Read the model definition and answer for the solid it produces. Units are mm, in the model's axes. Face numbers are marked on the shaded views. A direction names the side the tool comes from. Coordinates: 2 decimals unless noted, no trailing zeros. Order: outer loops, then holes, each group sorted by start corner. A loop starts at its lowest first (then second) coordinate and runs counter-clockwise, first axis right, second up. Notation, with made-up numbers: (76.25, 20.5) -> (126.25, 20.5) arc R20 cw to (126.25, 32.5) -> close; hole circle Ø10 at (-38, 54.25). An arc over 180 degrees is marked (long way). Answer as a JSON object with one key per item and string values. Group by question number.
1) Determine the mould class of the marked faces 3, 4, 5 and 6 for opening direction Z: released by +Z, released by -Z, zero draft, split by the parting line, or undercut.
2) Section A-A on x = 48 is taken. Determine the outline of the cut face in (y, z), and give its area (3 significant figures).
3) A tool of negligible diameter and unlimited length cuts with its end or side. For the marked faces 1 and 2, from which of +Z, -Z, +X, -X, +Y, -Y can it reach the whole face along a straight path? Write none if from no direction.
4) Section C-C on z = 3 is taken. Determine the outline of the cut face in (x, y), and give its area (3 significant figures).
5) Section B-B on y = 178.5 is taken. Determine the outline of the cut face in (x, z).
6) Given pin 1 (1 mm diameter, centred on y = 180.5, z = -15, fed in from -X); pin 2 (5 mm diameter, centred on y = 31.5, z = 26.5, fed in from +X); pin 3 (8 mm diameter, centred on x = 19, y = 131.5, fed in from +Z); pin 4 (4 mm diameter, centred on x = 12.7, y = 275, fed in from -Z), each flat-ended and moving along its own axis, determine where each tip first touches the part or whether it passes through.
7) Section D-D on x = 29.5 is taken. Determine the outline of the cut face in (y, z), and give its area (3 significant figures).
8) Consider L1, parallel to Y at x = 12.7, z = -11.5; L2, parallel to Z at x = 54, y = 95; L3, parallel to Y at x = 12.7, z = -3.5. Determine where each line is inside the solid, lowest interval first.
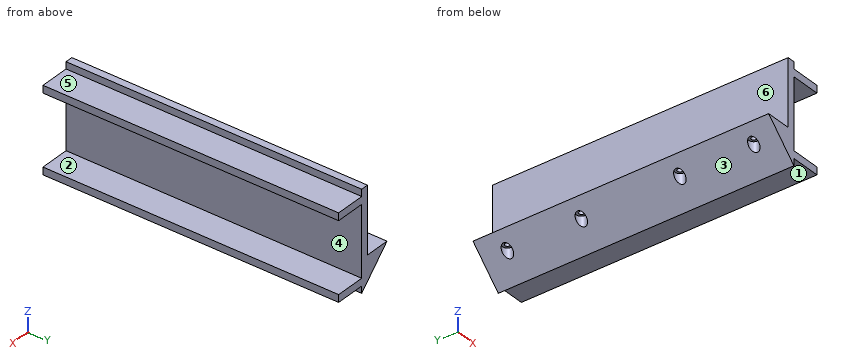
from build123d import *

# Parameters (mm, degrees)
BOSS_EXTRUDE1_DEPTH = 300
SKETCH3_R           = 2.5
CUT_EXTRUDE1_DEPTH  = 51
SKETCH4_R           = 5
CUT_EXTRUDE2_DEPTH  = 19


with BuildPart() as part:
    # Sketch1 → Boss-Extrude1 (new body)
    with BuildSketch(Plane(origin=(0, 0, 0), x_dir=(1, 0, 0), z_dir=(0, 1, 0))):
        Polygon((0, 0), (25.4, 0), (25.4, -50.8), (25.4, -67.1), (32.9, -67.1), (32.9, -60.1), (62.9, -60.1), (62.9, -52.6), (32.9, -52.6), (32.9, 18.4), (62.9, 18.4), (62.9, 25.9), (32.9, 25.9), (32.9, 32.9), align=None)
    extrude(amount=BOSS_EXTRUDE1_DEPTH)

    # Sketch3 → Cut-Extrude1 (cut)
    with BuildSketch(Plane(origin=(-25.9, 0, -25.9), x_dir=(1, 0, 0), z_dir=(0, 0, 1))):
        with Locations((38.6, 275)):
            Circle(SKETCH3_R)
        with Locations((38.6, 200)):
            Circle(SKETCH3_R)
        with Locations((38.6, 100)):
            Circle(SKETCH3_R)
        with Locations((38.6, 25)):
            Circle(SKETCH3_R)
    extrude(amount=CUT_EXTRUDE1_DEPTH, mode=Mode.SUBTRACT)

    # Sketch4 → Cut-Extrude2 (cut)
    with BuildSketch(Plane(origin=(0, 0, -25.9), x_dir=(-1, 0, 0), z_dir=(0, 0, -1))):
        with Locations((-12.7, 275)):
            Circle(SKETCH4_R)
        with Locations((-12.7, 200)):
            Circle(SKETCH4_R)
        with Locations((-12.7, 100)):
            Circle(SKETCH4_R)
        with Locations((-12.7, 25)):
            Circle(SKETCH4_R)
    extrude(amount=-CUT_EXTRUDE2_DEPTH, mode=Mode.SUBTRACT)


solid = part.part
Worked answers:
{
 "1": {"face 3": "released by -Z", "face 4": "undercut", "face 5": "released by +Z", "face 6": "zero draft"},
 "2": {"outline": "(0, -25.9) -> (300, -25.9) -> (300, -18.4) -> (0, -18.4) -> close; (0, 52.6) -> (300, 52.6) -> (300, 60.1) -> (0, 60.1) -> close", "area": "4,500 mm²"},
 "3": {"face 1": "-Z, +X, +Y, -Y", "face 2": "+X, +Y, -Y"},
 "4": {"outline": "(25.4, 0) -> (32.9, 0) -> (32.9, 300) -> (25.4, 300) -> close", "area": "2,250 mm²"},
 "5": {"outline": "(0, 0) -> (32.9, -32.9) -> (32.9, -25.9) -> (62.9, -25.9) -> (62.9, -18.4) -> (32.9, -18.4) -> (32.9, 52.6) -> (62.9, 52.6) -> (62.9, 60.1) -> (32.9, 60.1) -> (32.9, 67.1) -> (25.4, 67.1) -> (25.4, 0) -> close"},
 "6": {"pin 1": "stops at x = 14.5", "pin 2": "stops at x = 32.9", "pin 3": "stops at z = 0", "pin 4": "passes through"},
 "7": {"outline": "(0, -29.5) -> (300, -29.5) -> (300, 67.1) -> (0, 67.1) -> close", "area": "29,000 mm²"},
 "8": {"L1": "y = 0 to 20, 30 to 95, 105 to 195, 205 to 270, 280 to 300", "L2": "z = -25.9 to -18.4, 52.6 to 60.1", "L3": "y = 0 to 22.5, 27.5 to 97.5, 102.5 to 197.5, 202.5 to 272.5, 277.5 to 300"}
}
